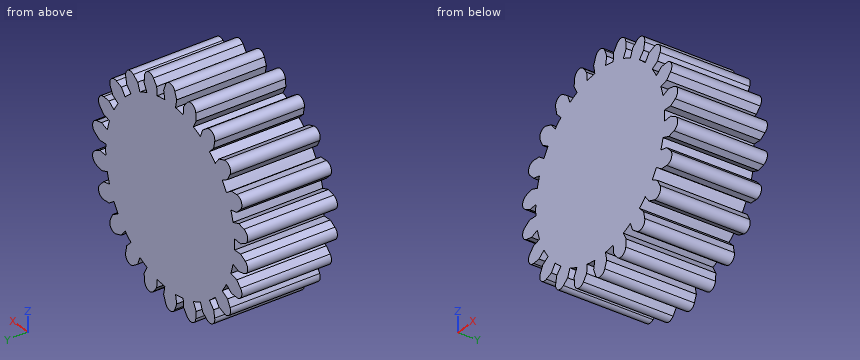
```python
from build123d import *

# Parameters (mm, degrees)
F0_R             = 25.4
F1_DEPTH         = 25.4
F4_DEPTH         = 25.4
F4_COPIES_COUNT  = 8
F4_COPIES_ANGLE  = 343.6356
F4_COPIES1_COUNT = 3
F4_COPIES1_ANGLE = 32.7272727273
F4_COPIES2_COUNT = 3
F4_COPIES2_ANGLE = 130.9088
F4_COPIES3_COUNT = 3
F4_COPIES3_ANGLE = 163.636
F4_COPIES4_COUNT = 3
F4_COPIES4_ANGLE = 229.0904


# Not quite as in the source:
# - a pattern or mirror of a feature is missing from the dataset's text; its kind, count and spacing are read off the source's solid


with BuildPart() as f1:
    # F0 (on Front) → F1 (new body)
    with BuildSketch(Plane.XZ):
        Circle(F0_R)
    extrude(amount=F1_DEPTH)

    # F3 (on Front) → F4 (join)
    with BuildSketch(Plane.XZ):
        with BuildLine():
            ThreePointArc((-2.0394499691, 25.0140055699), (0, 25.0970084039), (2.0394499691, 25.0140055699))
            Line((2.0394499691, 25.0140055699), (2.5789397816, 27.6699554159))
            Line((2.5789397816, 27.6699554159), (1.8071979284, 29.6250353105))
            ThreePointArc((1.8071979284, 29.6250353105), (0, 30.8545671303), (-1.8071979284, 29.6250353105))
            Line((-1.8071979284, 29.6250353105), (-2.5789397816, 27.6699554159))
            Line((-2.5789397816, 27.6699554159), (-2.0394499691, 25.0140055699))
        make_face()
    f4 = extrude(amount=F4_DEPTH)

    # F4_copies: F4 ×8 about axis
    f4_copies_axis = Axis((0, 0, 0), (0, -1, 0))
    for i in range(1, F4_COPIES_COUNT):
        add(f4.rotate(f4_copies_axis, i * F4_COPIES_ANGLE / (F4_COPIES_COUNT - 1)))

    # F4_copies1: F4 ×3 about axis
    f4_copies1_axis = Axis((0, 0, 0), (0, -1, 0))
    for i in range(1, F4_COPIES1_COUNT):
        add(f4.rotate(f4_copies1_axis, i * F4_COPIES1_ANGLE / (F4_COPIES1_COUNT - 1)))

    # F4_copies2: F4 ×3 about axis
    f4_copies2_axis = Axis((0, 0, 0), (0, -1, 0))
    for i in range(1, F4_COPIES2_COUNT):
        add(f4.rotate(f4_copies2_axis, i * F4_COPIES2_ANGLE / (F4_COPIES2_COUNT - 1)))

    # F4_copies3: F4 ×3 about axis
    f4_copies3_axis = Axis((0, 0, 0), (0, -1, 0))
    for i in range(1, F4_COPIES3_COUNT):
        add(f4.rotate(f4_copies3_axis, i * F4_COPIES3_ANGLE / (F4_COPIES3_COUNT - 1)))

    # F4_copies4: F4 ×3 about axis
    f4_copies4_axis = Axis((0, 0, 0), (0, -1, 0))
    for i in range(1, F4_COPIES4_COUNT):
        add(f4.rotate(f4_copies4_axis, i * F4_COPIES4_ANGLE / (F4_COPIES4_COUNT - 1)))

    # F4_copies5: F4 across plane
    add(f4.mirror(Plane(origin=(0, 0, 0), x_dir=(-0.7557528993, 0, -0.6548568968), z_dir=(0.6548568968, 0, -0.7557528993))))

    # F4_copies6: F4 across plane
    add(f4.mirror(Plane(origin=(0, 0, 0), x_dir=(-0.9594941358, 0, -0.2817285986), z_dir=(0.2817285986, 0, -0.9594941358))))

    # F4_copies7: F4 across plane
    add(f4.mirror(Plane(origin=(0, 0, 0), x_dir=(-1, 0, 1e-06), z_dir=(-1e-06, 0, -1))))

    # F4_copies8: F4 across plane
    add(f4.mirror(Plane(origin=(0, 0, 0), x_dir=(0.4154204975, 0, 0.9096294907), z_dir=(0.9096294907, 0, -0.4154204975))))

    # F4_copies9: F4 across plane
    add(f4.mirror(Plane(origin=(0, 0, 0), x_dir=(0.6548648109, 0, 0.7557460416), z_dir=(0.7557460416, 0, -0.6548648109))))

    # F4_copies10: F4 across plane
    add(f4.mirror(Plane(origin=(0, 0, 0), x_dir=(0.2817386464, 0, 0.9594911855), z_dir=(0.9594911855, 0, -0.2817386464))))


solid = f1.part
```
Could you check a few things on this model? Use its own coordinates, in mm. Round coordinates to 2 decimals unless told otherwise and drop trailing zeros. Loops run counter-clockwise (first coordinate to the right, second up) from the corner with the lowest first, then second, coordinate; pieces in that order, holes last.
Q1. For P1, Ø5, axis at x = -1.5, z = -20.5, coming from the +Y side; P2, Ø3, axis at y = -17.5, z = 23, coming from the -X side; P3, Ø6, axis at y = -18.5, z = 10, coming from the -X side; P4, Ø6, axis at x = -11, y = -5, coming from the -Z side, each with a flat end and sliding along its axis, tell me the tip position at first contact or that it passes through.
Q2. Please list where these lines run through material, in increasing order: L1, parallel to Z at x = -22, y = -12.5; L2, parallel to Z at x = -16, y = -1; L3, parallel to Z at x = 26, y = -19.5.
Q3. I want a section at A-A (x = -7.5). Write out the boundary of the cut face in (y, z), and give its area (3 significant figures).
Answer below:
1. P1: stops at y = 0
1. P2: stops at x = -17.57
1. P3: stops at x = -28.24
1. P4: stops at z = -29.68
2. L1: z = -20.87 to -15.83, -12.69 to 12.69, 15.83 to 20.87
2. L2: z = -26.23 to -20.72, -19.73 to 19.73, 20.72 to 26.23
2. L3: z = -13.94 to -9.09, -6.13 to -1.49, 1.49 to 6.13, 9.09 to 13.94
3. outline: (-25.4, -29.57) - (0, -29.57) - (0, 29.57) - (-25.4, 29.57) - close
3. area: 1,500 mm2
